Autodesk Inventor part; units mm, degrees
ref_plane "YZ Plane" through (0, 0, 0) normal (1, 0, 0) x (0, 1, 0)
ref_plane "XZ Plane" through (0, 0, 0) normal (0, 1, 0) x (-1, 0, 0)
ref_plane "XY Plane" through (0, 0, 0) normal (0, 0, 1) x (1, 0, 0)
sketch "スケッチ1" plane through (0, 0, 0) normal (0, 0, 1) x (1, 0, 0)
  line L0 (0, 0) -> (15, 0)
  line L1 (15, 0) -> (15, 15)
  line L2 (15, 15) -> (0, 15)
  line L3 (0, 15) -> (0, 0)
  dimension "d0" = 15
  dimension "d1" = 15
extrude "押し出し1" add sketch "スケッチ1" along normal blind 50
sketch "スケッチ3" plane through (0, 0, 0) normal (0, 0, -1) x (-1, 0, 0)
  line L0 (0, 15) -> (0, 0)
  line L1 (0, 0) -> (-15, 0)
  line L2 (-15, 0) -> (-15, 15)
  line L3 (-15, 15) -> (0, 15)
  line L4 (0, 15) -> (0, 0)
  dimension "d21" = 15
  dimension "d22" = 15
extrude "押し出し2" add sketch "スケッチ3" along normal blind 135
sketch "スケッチ4" plane through (0, 15, 50) normal (0, 1, 0) x (1, 0, 0)
  line L0 (15, 0) -> (15, 185)
  line L1 (15, 185) -> (0, 185)
  line L2 (0, 185) -> (0, 105)
  line L3 (0, 105) -> (15, 105)
  line L4 (15, 105) -> (15, 185)
  point P0 (0, 50)
  dimension "d25" = 15
  dimension "d26" = 80
extrude "押し出し3" cut sketch "スケッチ4" against normal blind 135
sketch "スケッチ5" plane through (15, 15, -55) normal (0, 0, -1) x (-1, 0, 0)
  line L0 (15, 0) -> (15, -15)
  line L1 (0, -15) -> (0, 0)
  line L2 (15, -15) -> (0, -15)
  line L3 (0, -15) -> (0, 0)
  line L4 (0, 0) -> (15, 0)
  line L5 (15, 0) -> (15, -15)
extrude "押し出し4" add sketch "スケッチ5" along normal blind 15
sketch "スケッチ8" plane through (15, 0, 50) normal (1, 0, 0) x (0, 0, -1)
  line L0 (120, 15) -> (120, 0)
  line L1 (120, 15) -> (0, 15)
  point P0 (50, 0)
  point P1 (90, 7.5)
  point P2 (80, 7.5)
  point P3 (70, 7.5)
  dimension "d54" = 30
  dimension "d55" = 7.5
  dimension "d56" = 7.5
  dimension "d57" = 7.5
  dimension "d58" = 10
  dimension "d59" = 10
hole "穴4" at (15, 7.5, -40) at (15, 7.5, -30) at (15, 7.5, -20) direction (-1, 0, 0) diameter 3.2 end through all
sketch "スケッチ9" plane through (15, 0, 50) normal (1, 0, 0) x (0, 0, -1)
  line L0 (0, 0) -> (0, 15)
  line L1 (0, 0) -> (120, 0)
  point P0 (50, 0)
  point P1 (10, 7.5)
  point P2 (20, 7.5)
  dimension "d67" = 10
  dimension "d68" = 10
  dimension "d69" = 7.5
  dimension "d70" = 7.5
hole "穴5" at (15, 7.5, 40) at (15, 7.5, 30) direction (-1, 0, 0) diameter 3.2 end through all
sketch "スケッチ10" plane through (15, 0, 50) normal (1, 0, 0) x (0, 0, -1)
  point P0 (50, 0)
sketch "スケッチ11" plane through (15, 0, 50) normal (1, 0, 0) x (0, 0, -1)
  line L0 (0, 0) -> (0, 15)
  line L1 (0, 0) -> (120, 0)
  point P0 (50, 0)
  point P1 (30, 7.5)
  dimension "d78" = 30
  dimension "d79" = 7.5
hole "穴6" at (15, 7.5, 20) direction (-1, 0, 0) diameter 3.2 end through all
sketch "スケッチ12" plane through (15, 15, -70) normal (0, 0, -1) x (-1, 0, 0)
  line L0 (0, 0) -> (0, -15)
  line L1 (0, 0) -> (15, 0)
  line L2 (15, 0) -> (15, -15)
  line L3 (15, -15) -> (0, -15)
  line L4 (0, -15) -> (0, 0)
extrude "押し出し5" add sketch "スケッチ12" along normal blind 5
sketch "スケッチ13" plane through (0, 15, 50) normal (0, 1, 0) x (1, 0, 0)
  line L0 (0, 125) -> (15, 125)
  point P0 (0, 50)
  point P1 (7.3304, 115)
  point P2 (7.5, 105)
  point P3 (7.5, 95)
  dimension "d89" = 10
  dimension "d90" = 10
  dimension "d91" = 10
hole "穴7" at (7.5, 15, -45) at (7.5, 15, -55) at (7.3304, 15, -65) direction (0, -1, 0) diameter 3.2 end through all
sketch "スケッチ14" plane through (0, 0, 50) normal (0, 0, 1) x (1, 0, 0)
  line L0 (1.5, 13.5) -> (13.5, 13.5)
  line L1 (13.5, 13.5) -> (13.5, 1.5)
  line L2 (13.5, 1.5) -> (1.5, 1.5)
  line L3 (1.5, 1.5) -> (1.5, 13.5)
  line L4 (15, 15) -> (0, 15)
  line L5 (0, 15) -> (0, 0)
  dimension "d99" = 12
  dimension "d100" = 12
  dimension "d101" = 1.5
  dimension "d102" = 1.5
extrude "押し出し6" cut sketch "スケッチ14" against normal blind 500
properties part number "射出_角柱10" material "アルミニウム 6061"
Design review of the part built by this model. Coordinates are the model's own, in mm. A direction names the side the tool comes from. Give positions to 0.01 mm unless a question says otherwise; leave off trailing zeros. Loops run counter-clockwise (first coordinate to the right, second up) from the corner with the lowest first, then second, coordinate; pieces in that order, holes last. Notation, with made-up numbers: (70.25, 9.25) -> (122.25, 9.25) arc R3 cw to (122.25, 14.25) -> close; hole circle Ø8 at (4.25, -18). An arc over 180 degrees is marked (long way). One line per item, written item: value.
Q1. We need section B-B on z = -55. Give the boundary of the cut face in (x, y).
Numbers:
outline: (0, 0) -> (5.9, 0) -> (5.9, 1.5) -> (1.5, 1.5) -> (1.5, 13.5) -> (5.9, 13.5) -> (5.9, 15) -> (0, 15) -> close; (9.1, 0) -> (15, 0) -> (15, 15) -> (9.1, 15) -> (9.1, 13.5) -> (13.5, 13.5) -> (13.5, 1.5) -> (9.1, 1.5) -> close
Q2. Machinability: for faces 1 (the flat face through (1, 8, -75)), 2 (the flat face through (1.5, 7, -12)), which of the approach directions +Z, -Z, +X, -X, +Y, -Y give a long, thin tool a straight path to every point of the face, cutting with its end or side? Answer none if there is none.
Numbers:
face 1: -Z, +X, -X, +Y, -Y
face 2: +Z, -Z
Q3. Draft analysis for pull direction Y (two halves, no side actions). For faces 3 (the flat face through (7, 0, -12)), 4 (the cylindrical face through (0.74, 8.47, -18.73)), 5 (the cylindrical face through (8.11, 14.24, -53.52)), state which applies: pulls with the +Y half, pulls with the -Y half, needs draft (parallel to the pull), parting line crosses it, or undercut.
Numbers:
face 3: pulls with the -Y half
face 4: undercut
face 5: needs draft
Q4. We need section D-D on z = -16. Give the boundary of the cut face in (x, y).
Numbers:
outline: (0, 0) -> (15, 0) -> (15, 15) -> (0, 15) -> close; hole (1.5, 1.5) -> (13.5, 1.5) -> (13.5, 13.5) -> (1.5, 13.5) -> close
Q5. For L1, parallel to Y at x = 6.75, z = -4; L2, parallel to Y at x = 14.2, z = 20, list the stretches that pass through material, from the lowest coordinate up.
Numbers:
L1: y = 0 to 1.5, 13.5 to 15
L2: y = 0 to 5.9, 9.1 to 15
Q6. We need section A-A on y = 10.5. Give the boundary of the cut face in (x, z).
Numbers:
outline: (0, -75) -> (1.5, -75) -> (1.5, 50) -> (0, 50) -> close; (13.5, -75) -> (15, -75) -> (15, 50) -> (13.5, 50) -> close
